Autodesk Inventor part; units mm, degrees
sketch "Sketch1" plane through (0, 0, 0) normal (0, 1, 0) x (-1, 0, 0)
  line L0 (165.1, 165.1) -> (-165.1, 165.1)
  line L1 (-165.1, 165.1) -> (-165.1, -165.1)
  line L2 (-165.1, -165.1) -> (165.1, -165.1)
  line L3 (165.1, -165.1) -> (165.1, 165.1)
  point P0 (0, 0)
  dimension "d0" = 330.2
  dimension "d1" = 330.2
  dimension "d2" = 165.1
  dimension "d3" = 165.1
extrude "Extrusion1" add sketch "Sketch1" along normal blind 279.4
sketch "Sketch2" plane through (-165.1, 0, 165.1) normal (0, 0, 1) x (1, 0, 0)
  line L0 (0, 279.4) -> (330.2, 279.4)
  line L1 (165.1, 279.4) -> (165.1, 247.65)
  arc A0 (207.6282, 242.4889) -> (122.5718, 242.4889) centre (165.1, 69.85) ccw
  line L2 (130.175, 196.85) -> (200.025, 196.85)
  line L3 (200.025, 196.85) -> (215.589, 223.8076)
  line L4 (130.175, 196.85) -> (114.611, 223.8076)
  arc A1 (122.5718, 242.4889) -> (114.611, 223.8076) centre (125.6096, 230.1576) ccw
  arc A2 (215.589, 223.8076) -> (207.6282, 242.4889) centre (204.5904, 230.1576) ccw
  point P0 (165.1, 0)
  dimension "d6" = 31.75
  dimension "d8" = 177.8
  dimension "d10" = 0
  dimension "d11" = 69.85
  dimension "d12" = 34.925
  dimension "d13" = 50.8
  dimension "d16" = 120
  dimension "d17" = 120
  dimension "d18" = 12.7
extrude "Extrusion2" cut sketch "Sketch2" against normal blind 25.4
sketch "Sketch3" plane through (165.1, 0, 165.1) normal (1, 0, 0) x (0, 0, -1)
  arc A0 (207.6282, 242.4889) -> (122.5718, 242.4889) centre (165.1, 69.85) ccw
  line L0 (130.175, 196.85) -> (200.025, 196.85)
  line L1 (200.025, 196.85) -> (215.589, 223.8076)
  line L2 (130.175, 196.85) -> (114.611, 223.8076)
  arc A1 (122.5718, 242.4889) -> (114.611, 223.8076) centre (125.6096, 230.1576) ccw
  arc A2 (215.589, 223.8076) -> (207.6282, 242.4889) centre (204.5904, 230.1576) ccw
  line L3 (0, 279.4) -> (330.2, 279.4)
  point P0 (165.1, 0)
  point P1 (165.1, 247.65)
  dimension "d21" = 177.8
  dimension "d22" = 69.85
  dimension "d23" = 50.8
  dimension "d24" = 120
  dimension "d25" = 120
  dimension "d26" = 12.7
  dimension "d27" = 31.75
  dimension "d28" = 34.925
extrude "Extrusion3" cut sketch "Sketch3" against normal blind 25.4
mirror "Mirror1" about plane through (0, 0, 0) normal (0, 0, 1) of "Extrusion2"
mirror "Mirror2" about plane through (0, 0, 0) normal (1, 0, 0) of "Extrusion3"
equation "\"d12\" = 0.5 * d11"
properties part number "POWER CUBE  1-9-2018"
Here's how the part is built. I have some questions about the finished solid (model axes, mm). A direction names the side the tool comes from. Give positions to 0.01 mm unless a question says otherwise; leave off trailing zeros. Order: outer loops, then holes, each group sorted by start corner. A loop starts at its lowest first (then second) coordinate and runs counter-clockwise, first axis right, second up. Notation, with made-up numbers: (51.5, -20.75) -> (59.5, -20.75) arc R17 ccw to (59.5, -2.75) -> close; hole circle Ø10 at (51, -31.5). An arc over 180 degrees is marked (long way). Use a Markdown table: item, result. Add a question column.
Item 1: Will this pin go through, and if not, where does the flat tip stop? pin 1 (1.5 mm diameter, centred on x = 19, y = 239.5, fed in from +Z).
Item 2: I need wall thicknesses on line 1 (Y direction, x = 2, z = 144.5). Which ranges of the line are inside material? Lowest first, please.
Item 3: Imagine slicing it at A-A on x = 0. Please give me the cut outline in (y, z).
Item 4: If we mould it in two halves opening along X, with no side actions, what happens to faces 5 (the face through (-42.816, 210.518, -152.578)), 6 (the face through (-139.7, 223, -1)), 7 (the face through (2, 0, 2))? For each: pulls with the +X half, pulls with the -X half, needs draft (parallel to the pull), parting line crosses it, or undercut.
Item 5: For faces 1 (the face through (-152.58, 247.65, 0.6)), 2 (the face through (-51.108, 235.287, 152.578)), 3 (the face through (152.578, 235.287, 51.108)), 4 (the face through (-0.6, 247.65, -152.58)), which set-ups out of +Z, -Z, +X, -X, +Y, -Y let a thin tool reach every point of the face, with its end or its side?
Item 6: Imagine slicing it at B-B on z = -6.5. Please give me the cut outline in (x, y), plus the area to 3 significant figures.
Data:
| question | item | result |
|---|---|---|
| 1 | pin 1 | stops at z = 139.7 |
| 2 | line 1 | y = 0 to 196.85, 247.64 to 279.4 |
| 3 | outline | (0, -165.1) -> (196.85, -165.1) -> (196.85, -139.7) -> (247.65, -139.7) -> (247.65, -165.1) -> (279.4, -165.1) -> (279.4, 165.1) -> (247.65, 165.1) -> (247.65, 139.7) -> (196.85, 139.7) -> (196.85, 165.1) -> (0, 165.1) -> close |
| 4 | face 5 | undercut |
| 4 | face 6 | pulls with the -X half |
| 4 | face 7 | needs draft |
| 5 | face 1 | -X |
| 5 | face 2 | +Z |
| 5 | face 3 | +X |
| 5 | face 4 | -Z |
| 6 | outline | (-165.1, 0) -> (165.1, 0) -> (165.1, 196.85) -> (139.7, 196.85) -> (139.7, 247.53) -> (165.1, 247.53) -> (165.1, 279.4) -> (-165.1, 279.4) -> (-165.1, 247.53) -> (-139.7, 247.53) -> (-139.7, 196.85) -> (-165.1, 196.85) -> close |
| 6 | area | 89,700 mm² |
